Autodesk Inventor part; units mm, degrees
ref_plane "YZ Plane" through (0, 0, 0) normal (1, 0, 0) x (0, 1, 0)
ref_plane "XZ Plane" through (0, 0, 0) normal (0, 1, 0) x (-1, 0, 0)
ref_plane "XY Plane" through (0, 0, 0) normal (0, 0, 1) x (1, 0, 0)
sketch "Sketch1" plane through (0, 0, 0) normal (0, 0, 1) x (1, 0, 0)
  line L0 (-15.4, 5.35) -> (15.4, 5.35)
  line L1 (15.4, 5.35) -> (15.4, -5.35)
  line L2 (15.4, -5.35) -> (-15.4, -5.35)
  line L3 (-15.4, -5.35) -> (-15.4, 5.35)
  line L4 (-15.4, 5.35) -> (15.4, -5.35) construction
  line L5 (15.4, 5.35) -> (-15.4, -5.35) construction
  line L6 (-15.4, 0.35) -> (15.4, 0.35) construction
  circle A0 centre (-12.5, 0.35) radius 1.25
  circle A1 centre (12.5, 0.35) radius 1.25
  line L7 (0, 5.35) -> (0, -5.35) construction
  circle A2 centre (-12.5, 0.35) radius 2.7424 construction
  line L8 (-13.8712, -2.025) -> (-11.1288, 2.725) construction
  line L9 (-13.8712, 2.725) -> (-11.1288, -2.025) construction
  line L10 (-9.7576, 0.35) -> (-15.2424, 0.35) construction
  line L11 (-11.1288, 2.725) -> (-13.8712, 2.725)
  line L12 (-13.8712, 2.725) -> (-15.2424, 0.35)
  line L13 (-15.2424, 0.35) -> (-13.8712, -2.025)
  line L14 (-13.8712, -2.025) -> (-11.1288, -2.025)
  line L15 (-11.1288, -2.025) -> (-9.7576, 0.35)
  line L16 (-9.7576, 0.35) -> (-11.1288, 2.725)
  line L17 (11.1288, 2.725) -> (13.8712, 2.725)
  line L18 (13.8712, 2.725) -> (15.2424, 0.35)
  line L19 (15.2424, 0.35) -> (13.8712, -2.025)
  line L20 (13.8712, -2.025) -> (11.1288, -2.025)
  line L21 (11.1288, -2.025) -> (9.7576, 0.35)
  line L22 (9.7576, 0.35) -> (11.1288, 2.725)
  line L23 (-7.5, 5.15) -> (7.5, 5.15)
  line L24 (7.5, 5.15) -> (9.5, 2.55)
  line L25 (9.5, 2.55) -> (8.5, -2.65)
  line L26 (8.5, -2.65) -> (6.75, -4.85)
  line L27 (6.75, -4.85) -> (-6.75, -4.85)
  line L28 (-6.75, -4.85) -> (-8.5, -2.65)
  line L29 (-8.5, -2.65) -> (-9.5, 2.55)
  line L30 (-9.5, 2.55) -> (-7.5, 5.15)
  point P0 (0, 0)
  dimension "d0" = 30.8
  dimension "d1" = 10.7
  dimension "d2" = 2.5
  dimension "d4" = 60
  dimension "d5" = 60
  dimension "d6" = 4.75
  dimension "d7" = 5
  dimension "d8" = 25
  dimension "d9" = 15
  dimension "d10" = 19
  dimension "d11" = 13.5
  dimension "d12" = 17
  dimension "d13" = 10
  dimension "d14" = 7.4
  dimension "d15" = 2.2
  dimension "d16" = 0.2
extrude "Extrusion1" add sketch "Sketch1" along normal blind 5 contours L16 L15 L14 L13 L12 L11 | L17 L18 L19 L20 L21 L22
extrude "Extrusion2" add sketch "Sketch1" along normal blind 6 contours L23 L24 L25 L26 L27 L28 L29 L30
extrude "Extrusion3" add sketch "Sketch1" against normal blind 9 contours L0 L1 L2 L3 | A0 | A1 | L16 L15 L14 L13 L12 L11 | L17 L18 L19 L20 L21 L22 | L23 L24 L25 L26 L27 L28 L29 L30
sketch "Sketch2" plane through (-15.4, 5.35, 0) normal (0, 1, 0) x (1, 0, 0)
  line L0 (0, 0) -> (30.8, 0)
  line L1 (30.8, 0) -> (30.8, 9)
  line L2 (0, 9) -> (30.8, 9)
  line L3 (0, 0) -> (0, 9)
  line L4 (15.4, 0) -> (15.4, 9) construction
  line L5 (0, 0) -> (0, 9)
  line L6 (0, 9) -> (6.9, 9)
  line L7 (6.9, 9) -> (6.9, 4.4)
  line L8 (6.9, 4.4) -> (0, 4.4)
  line L9 (0, 4.4) -> (0, 9)
  line L10 (30.8, 9) -> (0, 9)
  line L11 (30.8, 9) -> (23.9, 9)
  line L12 (23.9, 9) -> (23.9, 4.4)
  line L13 (23.9, 4.4) -> (30.8, 4.4)
  line L14 (30.8, 4.4) -> (30.8, 9)
  line L15 (6.9, 4.4) -> (23.9, 4.4) construction
  dimension "d23" = 17
  dimension "d24" = 4.4
extrude "Extrusion4" cut sketch "Sketch2" against normal blind 7.7 contours L3 L2 L7 L8 | L13 L12 L2 L1
sketch "Sketch3" plane through (0, 0, 6) normal (0, 0, 1) x (1, 0, 0)
  line L0 (-5, 2.5) -> (3.2977, 2.5) construction
  circle A0 centre (-5, 2.5) radius 1
  circle A1 centre (-2.5, 2.5) radius 1
  circle A2 centre (0, 2.5) radius 1
  circle A3 centre (2.5, 2.5) radius 1
  circle A4 centre (5, 2.5) radius 1
  line L1 (-6, 0) -> (3.7977, 0) construction
  circle A5 centre (-6, 0) radius 1
  circle A6 centre (-3.5, 0) radius 1
  circle A7 centre (-1, 0) radius 1
  circle A8 centre (1.5, 0) radius 1
  circle A9 centre (4, 0) radius 1
  line L2 (-5, -2.5) -> (3.1289, -2.5) construction
  circle A10 centre (-5, -2.5) radius 1
  circle A11 centre (-2.5, -2.5) radius 1
  circle A12 centre (0, -2.5) radius 1
  circle A13 centre (2.5, -2.5) radius 1
  circle A14 centre (5, -2.5) radius 1
  line L3 (0, 2.5) -> (0, -2.5) construction
  point P0 (0, 0)
  point P1 (0, 0)
  dimension "d27" = 2
  dimension "d30" = 2.5
  dimension "d39" = 2
  dimension "d40" = 2.5
  dimension "d50" = 2
  dimension "d51" = 2.5
  dimension "d53" = 2.5
  dimension "d54" = 2.5
extrude "Extrusion5" cut sketch "Sketch3" against normal blind 1
fillet "Fillet1" radius 3 8 edges at (-7.5, 5.15, 3) (-9.5, 2.55, 3) (-8.5, -2.65, 3) (-6.75, -4.85, 3) (6.75, -4.85, 3) (8.5, -2.65, 3) (9.5, 2.55, 3) (7.5, 5.15, 3)
sketch "Sketch4" plane through (0, 0, 0) normal (0, 1, 0) x (-1, 0, 0)
  line L0 (-15.4, -9) -> (15.4, -9)
  line L1 (15.4, -4.4) -> (15.4, -9)
  line L2 (-15.4, -9) -> (-15.4, -4.4)
  line L3 (15.4, -6.5) -> (13.9, -6.5)
  line L4 (13.9, -6.5) -> (13.9, -5)
  line L5 (10.9, -5) -> (10.9, -9)
  line L6 (10.9, -9) -> (15.4, -9)
  line L7 (15.4, -9) -> (15.4, -6.5)
  arc A0 (13.9, -5) -> (10.9, -5) centre (12.4, -5) ccw
  line L8 (8.5, -9) -> (-8.5, -9)
  line L9 (0, -9) -> (0, -5) construction
  arc A1 (10.9, -5) -> (13.9, -5) centre (12.4, -5) ccw construction
  line L10 (-15.4, -4.4) -> (-15.4, -9)
  line L11 (-15.4, -6.5) -> (-13.9, -6.5)
  line L12 (-13.9, -6.5) -> (-13.9, -5)
  line L13 (-10.9, -5) -> (-10.9, -9)
  line L14 (-10.9, -9) -> (-15.4, -9)
  line L15 (-15.4, -9) -> (-15.4, -6.5)
  arc A2 (-10.9, -5) -> (-13.9, -5) centre (-12.4, -5) ccw
  arc A3 (-13.9, -5) -> (-10.9, -5) centre (-12.4, -5) ccw construction
  point P0 (0, 0)
  dimension "d58" = 3
  dimension "d59" = 4
  dimension "d60" = 3
  dimension "d61" = 2.5
extrude "Extrusion6" cut sketch "Sketch4" against normal through all
fillet "Fillet2" radius 0.4 16 edges at (-7.3481, 4.8414, 6) (-8.5388, 3.7996, 6) (-9.2181, 2.4831, 6) (-8.9421, -0.3508, 6) (-8.4189, -2.6127, 6) (-7.8459, -3.4723, 6) (-6.6063, -4.5521, 6) (0, -4.85, 6) (6.6063, -4.5521, 6) (7.8459, -3.4723, 6) (8.4189, -2.6127, 6) (8.9421, -0.3508, 6) (9.2181, 2.4831, 6) (8.5388, 3.7996, 6) (7.3481, 4.8414, 6) (0, 5.15, 6)
equation "\"d5\" = d4"
equation "\"d54\" = d53"
properties part number "db15-connector-pcb"
Part model, mm, in its own coordinate system. A direction names the side the tool comes from. Give positions to 0.01 mm unless a question says otherwise; leave off trailing zeros. Loops run counter-clockwise (first coordinate to the right, second up) from the corner with the lowest first, then second, coordinate; pieces in that order, holes last. Notation, with made-up numbers: M 52.25,20.5 L 102.25,20.5 A30 ccw 102.25,50.5 Z; hole C 35,61.25 d11. An arc over 180 degrees is marked long. Put each result on its own line as item: value. Start each with the question number.
1) Saw through at B-B (x = -12.4). List the corners of the cut face in (y, z) (3 decimals), then the cut area to 3 significant figures.
2) Probe probe 1 along Z at (x, y) = (10.5, 1.75); probe 2 along Z at (x, y) = (1, 0); probe 3 along Y at (x, z) = (0.5, 0.25). List the from-to ranges inside material, lowest first.
3) Saw through at A-A (z = -7.5). List the corners of the cut face in (x, y), then the cut area to 3 significant figures.
4) Saw through at C-C (x = 12.5). List the corners of the cut face in (y, z) (3 decimals).
5) Flat gauge pins, fed straight in: pin 1 (6 mm diameter, centred on x = 11, y = 2.5, fed in from -Z); pin 2 (0.6 mm diameter, centred on x = 1.5, y = -0.5, fed in from +Z); pin 3 (1.5 mm diameter, centred on x = -12.5, y = 0.35, fed in from -Z); pin 4 (0.8 mm diameter, centred on x = -14.5, y = -4.5, fed in from -Z). Where does each tip first touch, or does it go through?
6) Pull direction Y, two halves, no side cores. Call faces 1 (the flat face through (10.9, -4, -7)), 2 (the flat face through (-3, -2, 5)), 3 (the flat face through (14.566, -0.821, 2.465)): +Y half, -Y half, draft (parallel to the pull), parting line (faces both ways), or undercut.
7) 3-axis set-ups, long thin cutter, end or side, ignore diameter. For faces 4 (the flat face through (0, -2, 5)), 5 (the cylindrical face through (6.59, -4.56, 2.84)), 6 (the flat face through (-13.9, -4, -6)): which of +Z, -Z, +X, -X, +Y, -Y reach the whole face in a straight line?
Numbers:
1. outline: M -5.35,-3.5 L 0,-3.5 L 0,-4.4 L 5.35,-4.4 L 5.35,0 L 2.725,0 L 2.725,5 L 1.596,5 L 1.596,0 L -0.896,0 L -0.896,5 L -2.025,5 L -2.025,0 L -5.35,0 Z
1. area: 53.6 mm^2
2. probe 1: -4.4 to 0
2. probe 2: -9 to 5
2. probe 3: -4.85 to 5.15
3. outline: M -10.9,-5.35 L 10.9,-5.35 L 10.9,-2.35 L 8.5,-2.35 L 8.5,5.35 L -8.5,5.35 L -8.5,-2.35 L -10.9,-2.35 Z
3. area: 196 mm^2
4. outline: M -5.35,-3.503 L 0,-3.503 L 0,-4.4 L 5.35,-4.4 L 5.35,0 L 2.725,0 L 2.725,5 L 1.6,5 L 1.6,0 L -0.9,0 L -0.9,5 L -2.025,5 L -2.025,0 L -5.35,0 Z
5. pin 1: z = -9
5. pin 2: z = 5
5. pin 3: z = -4.4
5. pin 4: z = -6.5
6. face 1: draft
6. face 2: undercut
6. face 3: -Y half
7. face 4: +Z
7. face 5: +Z, +X, -Y
7. face 6: -Z, +Y, -Y
